```python
from build123d import *

# Parameters (mm, degrees)
SALIENTE_EXTRUIR1_DEPTH = 25
REDONDEO1_R             = 5
VACIADO1_T              = -2
SALIENTE_EXTRUIR2_DEPTH = 2.5
REDONDEO3_R             = 1
CROQUIS4_R              = 2
CORTAR_EXTRUIR1_DEPTH   = 43.193943257
CORTAR_EXTRUIR2_DEPTH   = 10


with BuildPart() as part:
    # Croquis1 → Saliente-Extruir1 (new body)
    with BuildSketch(Plane(origin=(0, 0, 0), x_dir=(0, 0, -1), z_dir=(1, 0, 0))):
        with BuildLine():
            Line((0, 0), (20, 0))
            Line((20, 0), (20, 20))
            Line((20, 20), (0, 20))
            ThreePointArc((0, 20), (-10, 10), (0, 0))
        make_face()
    extrude(amount=SALIENTE_EXTRUIR1_DEPTH)

    # Redondeo1
    redondeo1_edges = [part.edges().sort_by_distance(p)[0] for p in [
        (25, 20, -10),
        (25, 10, 10),
        (0, 20, -10),
        (0, 0, -10),
        (0, 10, 10),
        (25, 0, -10),
    ]]
    fillet(redondeo1_edges, radius=REDONDEO1_R)

    # Vaciado1
    vaciado1_openings = [part.faces().sort_by_distance(p)[0] for p in [
        (12.5, 10, -20),
    ]]
    offset(amount=VACIADO1_T, openings=vaciado1_openings, kind=Kind.INTERSECTION)


with BuildPart() as saliente_extruir2_tool:
    # Croquis3 → Saliente-Extruir2 (new, symmetric)
    with BuildSketch(Plane(origin=(12.5, 0, 0), x_dir=(0, 0, -1), z_dir=(1, 0, 0))):
        with BuildLine():
            Line((20, 20), (20, 33.990128519))
            Line((20, 33.990128519), (11.304943529, 33.990128519))
            ThreePointArc((11.304943529, 33.990128519), (7.637753489, 25.384236828), (-0.012060129, 20))
            Line((-0.012060129, 20), (20, 20))
        make_face()
    extrude(amount=SALIENTE_EXTRUIR2_DEPTH, both=True)


with BuildPart() as part_1:
    add(part.part)


with BuildPart() as part_2:
    # Saliente-Extruir2: joined with saliente_extruir2_tool
    add(part_1.part.fuse(saliente_extruir2_tool.part, tol=0.00001))

    # Redondeo3
    redondeo3_edges = [part_2.edges().sort_by_distance(p)[0] for p in [
        (15, 33.990128519, -15.652471765),
        (15, 26.99506426, -20),
        (15, 25.384236828, -7.637753489),
        (10, 26.99506426, -20),
        (10, 25.384236828, -7.637753489),
        (10, 33.990128519, -15.652471765),
    ]]
    fillet(redondeo3_edges, radius=REDONDEO3_R)

    # Croquis4 → Cortar-Extruir1 (cut, through all)
    with BuildSketch(Plane(origin=(15, 0, 0), x_dir=(0, 0, -1), z_dir=(1, 0, 0))):
        with Locations((15.652471765, 29.990128519)):
            Circle(CROQUIS4_R)
    extrude(amount=-CORTAR_EXTRUIR1_DEPTH, mode=Mode.SUBTRACT)

    # Croquis5 → Cortar-Extruir2 (cut)
    with BuildSketch(Plane(origin=(15, 0, 0), x_dir=(0, 0, -1), z_dir=(1, 0, 0))):
        with BuildLine():
            Line((-7.217046024, 20), (0, 20))
            ThreePointArc((0, 20), (5.136167379, 22.500777517), (9.478440599, 26.212753651))
            ThreePointArc((9.478440599, 26.212753651), (11.166757122, 29.464653871), (12.164903517, 32.990128519))
            Line((12.164903517, 32.990128519), (15.652471765, 32.990128519))
            Line((15.652471765, 32.990128519), (19, 32.990128519))
            Line((19, 32.990128519), (19, 25.180898104))
            ThreePointArc((19, 25.180898104), (19.419701922, 22.57495018), (20, 20))
            Line((20, 20), (25.571513897, 20))
            Line((25.571513897, 20), (25.571513897, 39.781584786))
            Line((25.571513897, 39.781584786), (-7.217046024, 39.781584786))
            Line((-7.217046024, 39.781584786), (-7.217046024, 20))
        make_face()
        with BuildLine():
            ThreePointArc((12.164903517, 32.990128519), (11.166757122, 29.464653871), (9.478440599, 26.212753651))
            ThreePointArc((9.478440599, 26.212753651), (11.398291791, 28.648352134), (12.965556832, 31.324477852))
            ThreePointArc((12.965556832, 31.324477852), (14.071814939, 32.539937139), (15.652471765, 32.990128519))
            Line((15.652471765, 32.990128519), (12.164903517, 32.990128519))
        make_face()
        with BuildLine():
            ThreePointArc((18.652159682, 30.033399776), (18.756747814, 27.602179034), (19, 25.180898104))
            Line((19, 25.180898104), (19, 32.990128519))
            Line((19, 32.990128519), (15.652471765, 32.990128519))
            ThreePointArc((15.652471765, 32.990128519), (17.758437841, 32.12669279), (18.652159682, 30.033399776))
        make_face()
    extrude(amount=-CORTAR_EXTRUIR2_DEPTH, mode=Mode.SUBTRACT)


solid = part_2.part
```
Can you work these out from the model? Positions are in its coordinate system, mm. A direction names the side the tool comes from. Coordinates: 2 decimals unless noted, no trailing zeros. Write each loop counter-clockwise with the first axis right and the second up, starting at its lowest first coordinate (ties: lowest second). Pieces come first, ordered by that corner, then holes. Notation, with made-up numbers: M 8.25,21 L 64.25,21 A22 ccw 64.25,42 Z; hole C 49.5,-30 d8. An arc over 180 degrees is marked long. Answer as CSV lines item,"result".
Item 1: Imagine slicing it at A-A on z = -11. List the corners of the cut face in (x, y) for me, plus the area to 3 significant figures.
Geometry results:
outline,"M 0,5 A5 ccw 5,0 L 20,0 A5 ccw 25,5 L 25,15 A5 ccw 20,20 L 15,20 L 15,28.08 L 10,28.08 L 10,20 L 5,20 A5 ccw 0,15 Z; hole M 2,5 A3 ccw 5,2 L 20,2 A3 ccw 23,5 L 23,15 A3 ccw 20,18 L 5,18 A3 ccw 2,15 Z"
area,"191 mm2"
Item 2: Imagine slicing it at B-B on x = 17. List the corners of the cut face in (y, z) for me, plus the area to 3 significant figures.
Geometry results:
outline,"M 0,-20 L 2,-20 L 2,0 A8 cw 18,0 L 18,-20 L 20,-20 L 20,0 A10 ccw 0,0 Z"
area,"137 mm2"
Item 3: On a 3-axis mill with a long thin cutter (end or side, diameter ignored), from which of +Z, -Z, +X, -X, +Y, -Y can I reach the whole of each face in a straight line? I mean faces 1 (the cylindrical face through (12, 10, 10)), 2 (the flat face through (23, 10, -7)). Say none if no direction works.
Geometry results:
face 1,"+Z, +X, -X"
face 2,"-Z"
Item 4: I'm going to push flat-ended pins straight in: P1, Ø5, axis at y = 29.99, z = -15.65, coming from the +X side; P2, Ø12, axis at y = 17.5, z = -11.5, coming from the +X side; P3, Ø10.5, axis at y = 27.5, z = -10, coming from the -X side; P4, Ø3, axis at x = 17, z = -6.5, coming from the +Y side. Where does each tip first touch, or does it pass through?
Geometry results:
P1,"stops at x = 15"
P2,"stops at x = 25"
P3,"stops at x = 10"
P4,"stops at y = 20"
Item 5: We'd pull the mould along X, two halves only. Please class faces 3 (the cylindrical face through (22.1, 17.14, -9.86)), 4 (the flat face through (15, 25, -14)), 5 (the flat face through (8, 20, -10)): +X half, -X half, draft (parallel to the pull), parting line (faces both ways), or undercut.
Geometry results:
face 3,"undercut"
face 4,"+X half"
face 5,"draft"
Item 6: Please list where these lines run through material, in increasing order: line 1 along X through (y, z) = (5, 0.5); line 2 along Y through (x, z) = (20, -6); line 3 along Y through (x, z) = (10.5, -17).
Geometry results:
line 1,"x = 0 to 2, 23 to 25"
line 2,"y = 0 to 2, 18 to 20"
line 3,"y = 0 to 2, 18 to 28.51, 31.47 to 32.67"
